```python
from build123d import *

# Parameters (mm, degrees)
BOX015_W               = 12
BOX015_H               = 10
BOX015_DEPTH           = 12
ARRAY001_X_COUNT       = 4
ARRAY001_X_PITCH       = 14.4
ARRAY001_Z_COUNT       = 2
ARRAY001_Z_PITCH       = 14
BOX014_W               = 60
BOX014_H               = 10
BOX014_DEPTH           = 30
CUT002_PLACEMENT_ANGLE = 90


with BuildPart() as obj1:
    # Box015 → Box015 (new body)
    with BuildSketch(Plane.XY):
        with Locations((6, 5)):
            Rectangle(BOX015_W, BOX015_H)
    extrude(amount=BOX015_DEPTH)

    # Array001 X: obj1 ×4


with BuildPart() as obj1_1:
    add(obj1.part)
    with Locations(*[(i * ARRAY001_X_PITCH, 0, 0) for i in range(1, ARRAY001_X_COUNT)]):
        add(obj1.part)

    # Array001 Z: obj1_2


with BuildPart() as obj1_2:
    add(obj1_1.part)
    with Locations(*[(0, 0, i * ARRAY001_Z_PITCH) for i in range(1, ARRAY001_Z_COUNT)]):
        add(obj1_1.part)


with BuildPart() as obj1_3:
    # Array001 placement: moved
    add(obj1_2.part.moved(Location((27.4, 91, 2))))


with BuildPart() as obj2:
    # Box014 → Box014 (new body)
    with BuildSketch(Plane(origin=(25, 90, 0), x_dir=(1, 0, 0), z_dir=(0, 0, 1))):
        with Locations((30, 5)):
            Rectangle(BOX014_W, BOX014_H)
    extrude(amount=BOX014_DEPTH)

    # Cut002: cut obj1
    add(obj1_3.part, mode=Mode.SUBTRACT)


with BuildPart() as obj2_1:
    # Cut002 placement: moved
    add(obj2.part.moved(Location((210, 0, 97))).rotate(Axis((210, 0, 97), (0, 0, 1)), CUT002_PLACEMENT_ANGLE))


solid = obj2_1.part
```
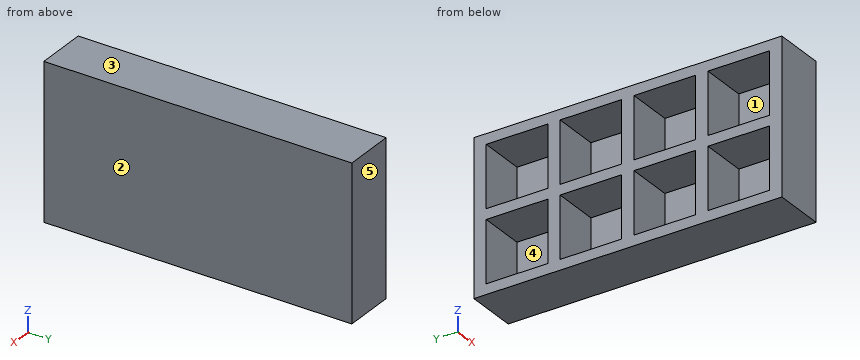
The listing builds one solid part. Answer for the finished solid, in the listing's coordinates (mm). Face numbers are marked on the shaded views. A direction names the side the tool comes from. Round coordinates to 2 decimals unless told otherwise and drop trailing zeros. Loops run counter-clockwise (first coordinate to the right, second up) from the corner with the lowest first, then second, coordinate; pieces in that order, holes last. Notation, with made-up numbers: (89.25, 62) - (132.25, 62) arc R21 ccw to (132.25, 70) - close; hole circle Ø4 at (13.5, 59). An arc over 180 degrees is marked (long way). Return JSON: item names as keys, results as strings. Group by question number.
1. Which of the six approach directions +Z, -Z, +X, -X, +Y, -Y give full straight-line access (tool end or side, diameter ignored) to the marked faces 1 and 2?
2. The part is cut by section B-B on y = 77.5. Determine the outline of the cut face in (x, z).
3. The mould has two halves that part along Z. Classify the marked faces 3, 4 and 5: pulls with the +Z half, pulls with the -Z half, needs draft (parallel to the pull), parting line crosses it, or undercut.
4. The part is cut by section A-A on z = 123.5. Determine the outline of the cut face in (x, y), then the cut area to 3 significant figures.
5. This flat-tipped pin is pushed along its axis until it touches: P1, Ø6, axis at y = 78.5, z = 102.5, coming from the -X side. Where does it stop, or does it pass through?
6. Consider probe 1 along Y at (x, z) = (114.5, 120.25); probe 2 along Z at (x, y) = (115.25, 79); probe 3 along X at (y, z) = (73, 119). Determine where each line is inside the solid, lowest interval first.
7. The part is cut by section C-C on x = 115. State how many separate pieces and enclosed holes the cut face has, then the cut area to 3 significant figures.
Resolved:
{
 "1": {"face 1": "-X", "face 2": "+Z, -Z, +X, +Y, -Y"},
 "2": {"outline": "(110, 97) - (120, 97) - (120, 127) - (110, 127) - (110, 125) - (119, 125) - (119, 113) - (110, 113) - (110, 111) - (119, 111) - (119, 99) - (110, 99) - close"},
 "3": {"face 3": "pulls with the +Z half", "face 4": "undercut", "face 5": "needs draft"},
 "4": {"outline": "(110, 25) - (120, 25) - (120, 85) - (110, 85) - (110, 82.6) - (119, 82.6) - (119, 70.6) - (110, 70.6) - (110, 68.2) - (119, 68.2) - (119, 56.2) - (110, 56.2) - (110, 53.8) - (119, 53.8) - (119, 41.8) - (110, 41.8) - (110, 39.4) - (119, 39.4) - (119, 27.4) - (110, 27.4) - close", "area": "168 mm²"},
 "5": {"P1": "stops at x = 119"},
 "6": {"probe 1": "y = 25 to 27.4, 39.4 to 41.8, 53.8 to 56.2, 68.2 to 70.6, 82.6 to 85", "probe 2": "z = 97 to 99, 111 to 113, 125 to 127", "probe 3": "x = 119 to 120"},
 "7": {"separate pieces": "1", "enclosed holes": "8", "area": "648 mm²"}
}
